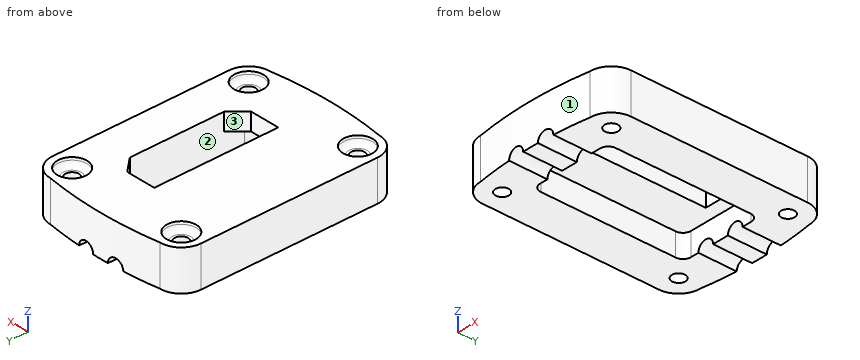
from build123d import *

# Parameters (mm, degrees)
F0_R      = 5.5
F0_R_2    = 2.5
F1_DEPTH  = 15
F2_R      = 5.5
F2_R_2    = 2.5
F3_DEPTH  = 3
F7_DEPTH  = 16
F9_DEPTH  = 8.5
F10_R     = 2
F4_R      = 3
F11_DEPTH = 43


# Not quite as in the source:
# - a feature names something its author has since deleted; it is built from what else it names


with BuildPart() as f1:
    # F0 (on Top) → F1 (new body)
    with BuildSketch(Plane.XY):
        with BuildLine():
            Line((30.2499662921, -32.75), (30.2499662921, 32.75))
            ThreePointArc((30.2499662921, 32.75), (27.9068205416, 38.4068542495), (22.2499662921, 40.75))
            ThreePointArc((22.2499662921, 40.75), (0, 42.5), (-22.2499662921, 40.75))
            ThreePointArc((-22.2499662921, 40.75), (-27.9068192027, 38.4068555884), (-30.2499662921, 32.7500037869))
            Line((-30.2499662921, 32.7500037869), (-30.2499662921, -32.75))
            ThreePointArc((-30.2499662921, -32.75), (-27.9068205416, -38.4068542495), (-22.2499662921, -40.75))
            ThreePointArc((-22.2499662921, -40.75), (0, -42.5), (22.2499662921, -40.75))
            ThreePointArc((22.2499662921, -40.75), (27.9068205416, -38.4068542495), (30.2499662921, -32.75))
        make_face()
        with Locations((-22.2499662921, -32.75)):
            Circle(F0_R, mode=Mode.SUBTRACT)
        with Locations((22.2499662921, -32.75)):
            Circle(F0_R, mode=Mode.SUBTRACT)
        with Locations((-22.2499662921, 32.75)):
            Circle(F0_R, mode=Mode.SUBTRACT)
        with Locations((22.2499662921, 32.75)):
            Circle(F0_R, mode=Mode.SUBTRACT)
        with Locations((-22.2499662921, 32.75)):
            Circle(F0_R)
        with Locations((-22.2499662921, 32.75)):
            Circle(F0_R_2, mode=Mode.SUBTRACT)
        with Locations((22.2499662921, 32.75)):
            Circle(F0_R)
        with Locations((22.2499662921, 32.75)):
            Circle(F0_R_2, mode=Mode.SUBTRACT)
        with Locations((22.2499662921, -32.75)):
            Circle(F0_R)
        with Locations((22.2499662921, -32.75)):
            Circle(F0_R_2, mode=Mode.SUBTRACT)
        with Locations((-22.2499662921, -32.75)):
            Circle(F0_R)
        with Locations((-22.2499662921, -32.75)):
            Circle(F0_R_2, mode=Mode.SUBTRACT)
    extrude(amount=F1_DEPTH)

    # F2 (on face) → F3 (cut)
    with BuildSketch(Plane.XY.offset(15)):
        with Locations((-22.2499662921, 32.75)):
            Circle(F2_R)
        with Locations((-22.2499662921, 32.75)):
            Circle(F2_R_2, mode=Mode.SUBTRACT)
        with Locations((22.2499662921, 32.75)):
            Circle(F2_R)
        with Locations((22.2499662921, 32.75)):
            Circle(F2_R_2, mode=Mode.SUBTRACT)
        with Locations((22.2499662921, -32.75)):
            Circle(F2_R)
        with Locations((22.2499662921, -32.75)):
            Circle(F2_R_2, mode=Mode.SUBTRACT)
        with Locations((-22.2499662921, -32.75)):
            Circle(F2_R)
        with Locations((-22.2499662921, -32.75)):
            Circle(F2_R_2, mode=Mode.SUBTRACT)
    extrude(amount=-F3_DEPTH, mode=Mode.SUBTRACT)

    # F6 (on Top) + F5 (on Top) → F7 (cut)
    with BuildSketch(Plane.XY):
        Polygon((-0.5, 23), (-0.5, 0), (-0.5, -23), (10.5, -23), (15.5, -17.5), (15.5, 0), (15.5, 17.5), (10.5, 23), align=None)
    with BuildSketch(Plane.XY):
        Polygon((10.5, 22.5), (0, 22.5), (0, -22.5), (10.5, -22.5), (15, -17.5), (15, 17.5), align=None)
    extrude(amount=F7_DEPTH, mode=Mode.SUBTRACT)

    # F8 (on face) → F9 (cut)
    with BuildSketch(Plane.XY):
        with BuildLine():
            Line((10.5, 23), (15.5, 17.5))
            Line((15.5, 17.5), (15.5, 25))
            ThreePointArc((15.5, 25), (14.6213203436, 27.1213203436), (12.5, 28))
            Line((12.5, 28), (-12, 28))
            ThreePointArc((-12, 28), (-14.1213203436, 27.1213203436), (-15, 25))
            Line((-15, 25), (-15, -25))
            ThreePointArc((-15, -25), (-14.1213203436, -27.1213203436), (-12, -28))
            Line((-12, -28), (12.5, -28))
            ThreePointArc((12.5, -28), (14.6213203436, -27.1213203436), (15.5, -25))
            Line((15.5, -25), (15.5, -17.5))
            Line((15.5, -17.5), (10.5, -23))
            Line((10.5, -23), (-0.5, -23))
            Line((-0.5, -23), (-0.5, 23))
            Line((-0.5, 23), (10.5, 23))
        make_face()
    extrude(amount=F9_DEPTH, mode=Mode.SUBTRACT)

    # F10
    f10_edges = [f1.edges().sort_by_distance(p)[0] for p in [
        (-27.749966, -32.75, 12),
        (16.749966, -32.75, 12),
        (-27.749966, 32.75, 12),
        (16.749966, 32.75, 12),
    ]]
    fillet(f10_edges, radius=F10_R)

    # F4 (on Front) → F11 (cut, symmetric)
    with BuildSketch(Plane.XZ):
        with Locations((6, 0)):
            Circle(F4_R)
        with Locations((-6, 0)):
            Circle(F4_R)
    extrude(amount=F11_DEPTH, both=True, mode=Mode.SUBTRACT)


solid = f1.part
The listing builds one solid part. Answer for the finished solid, in the listing's coordinates (mm). Face numbers are marked on the shaded views. A direction names the side the tool comes from. Give positions to 0.01 mm unless a question says otherwise; leave off trailing zeros. Write each loop counter-clockwise with the first axis right and the second up, starting at its lowest first coordinate (ties: lowest second). Pieces come first, ordered by that corner, then holes.
1) Given P1, Ø4, axis at x = 4, z = 4, coming from the -Y side; P2, Ø7.5, axis at x = -23.5, y = -33, coming from the +Z side; P3, Ø2, axis at x = -5, y = -21.5, coming from the -Z side; P4, Ø2, axis at x = 21.5, y = -32.5, coming from the +Z side, each flat-ended and moving along its own axis, determine where each tip first touches the part or whether it passes through.
2) Section A-A (y = 15) is taken. Write down the section's boundary in (x, z).
3) Section C-C (x = 4) is taken. Write down the section's boundary in (y, z).
4) Find the intervals of material crossed by L1, parallel to X at y = -17, z = 7; L2, parallel to X at y = 4.5, z = 14; L3, parallel to Y at x = -23.5, z = 7.5, in increasing order.
5) Section D-D (x = -7.5) is taken. Write down the section's boundary in (y, z), and give its area (3 significant figures).
6) Section B-B (z = 7.25) is taken. Write down the section's boundary in (x, y), and give its area (3 significant figures).
7) A tool of negligible diameter and unlimited length cuts with its end or side. For the marked faces 1, 2 and 3, from which of +Z, -Z, +X, -X, +Y, -Y can it reach the whole face along a straight path? Write none if from no direction.
Response:
1. P1: stops at y = -42.49
1. P2: stops at z = 12.71
1. P3: stops at z = 8.5
1. P4: passes through
2. outline: (-30.25, 0) - (-15, 0) - (-15, 8.5) - (-0.5, 8.5) - (-0.5, 15) - (-30.25, 15) - close; (15.5, 0) - (30.25, 0) - (30.25, 15) - (15.5, 15) - close
3. outline: (-42.44, 2.24) - (-28, 2.24) - (-28, 8.5) - (-23, 8.5) - (-23, 15) - (-42.44, 15) - close; (23, 8.5) - (28, 8.5) - (28, 2.24) - (42.44, 2.24) - (42.44, 15) - (23, 15) - close
4. L1: x = -30.25 to -15, 15.5 to 30.25
4. L2: x = -30.25 to -0.5, 15.5 to 30.25
4. L3: y = -40.65 to -34.92, -30.58 to 30.58, 34.92 to 40.65
5. outline: (-42.3, 2.6) - (-28, 2.6) - (-28, 8.5) - (28, 8.5) - (28, 2.6) - (42.3, 2.6) - (42.3, 15) - (-42.3, 15) - close
5. area: 719 mm2
6. outline: (-30.25, -32.75) arc R8 ccw to (-22.25, -40.75) arc R142.32 ccw to (22.25, -40.75) arc R8 ccw to (30.25, -32.75) - (30.25, 32.75) arc R8 ccw to (22.25, 40.75) arc R142.32 ccw to (-22.25, 40.75) arc R8 ccw to (-30.25, 32.75) - close; hole circle Ø5 at (-22.25, -32.75); hole circle Ø5 at (-22.25, 32.75); hole (-15, -25) arc R3 ccw to (-12, -28) - (12.5, -28) arc R3 ccw to (15.5, -25) - (15.5, 25) arc R3 ccw to (12.5, 28) - (-12, 28) arc R3 ccw to (-15, 25) - close; hole circle Ø5 at (22.25, -32.75); hole circle Ø5 at (22.25, 32.75)
6. area: 3,200 mm2
7. face 1: +Z, -Z, -Y
7. face 2: -Z
7. face 3: +Z, -Z
